Source: CAD feature listing. Evaluate the final solid. Frame: model axes, mm. A direction names the side the tool comes from. Give positions to 0.01 mm unless a question says otherwise; leave off trailing zeros. Loops run counter-clockwise (first coordinate to the right, second up) from the corner with the lowest first, then second, coordinate; pieces in that order, holes last. Notation, with made-up numbers: (-13.5, 88) - (33.5, 88) arc R21 ccw to (33.5, 105) - close; hole circle Ø6 at (66, -5.75). An arc over 180 degrees is marked (long way). Put each result on its own line as item: value.
Solid Edge part; units mm, degrees
sketch "Sketch1" plane through (0, 0, 0) normal (0, -1, 0) x (1, 0, 0)
  line L0 (4.25, 5) -> (4.25, 0)
  line L1 (4.25, 0) -> (2.85, 0)
  line L2 (2.85, 0) -> (2.5, -0.6062)
  line L3 (2.5, -0.6062) -> (2.5, -40)
  line L4 (2.5, -40) -> (0, -40)
  line L5 (2.3, 2.5) -> (0, 1.1721)
  line L6 (2.3, 5) -> (2.3, 2.5)
  line L7 (4.25, 5) -> (2.3, 5)
revolve "RevolvedProtrusion1" add sketch "Sketch1" angle 360 about axis through (0, 0, -6) along (0, 0, 1)
cosmetic_thread "Thread1"
chamfer "Chamfer_1" distance 0.25 angle 45 1 edges at (-2.5, 0, -40)
fillet "Round_1" radius 0.3 2 edges at (-4.25, 0, 0) (-4.25, 0, 5)
sketch "Sketch2" plane through (0, 0, 5) normal (0, 0, 1) x (0, 1, 0)
  line L0 (-2.3, 1.3279) -> (-2.3, -1.3279)
  line L1 (0, -2.6558) -> (-2.3, -1.3279)
  line L2 (2.3, -1.3279) -> (0, -2.6558)
  line L3 (2.3, 1.3279) -> (2.3, -1.3279)
  line L4 (0, 2.6558) -> (2.3, 1.3279)
  line L5 (-2.3, 1.3279) -> (0, 2.6558)
extrude "Cutout1" cut sketch "Sketch2" against normal up to vertex (2.5 mm away)
properties part number "STD-DIN912-M5x40x8.8" material "Galvanized steel"
1) Material intervals for line 1 along Z through (x, y) = (2.75, 2.25); line 2 along Y through (x, z) = (0, 2); line 3 along X through (y, z) = (1, -15), sorted ascending. Write a range as [from, to].
Check result:
line 1: [0, 5]
line 2: [-4.25, -1.43], [1.43, 4.25]
line 3: [-2.29, 2.29]
2) Pin query (flat end, axial travel): P1, Ø2, axis at x = 1, z = -24.5, coming from the -Y side; P2, Ø1.3, axis at x = -1, y = 1.5, coming from the +Z side; P3, Ø1.3, axis at x = -1, y = -2, coming from the +Z side; P4, Ø1.5, axis at x = 0, y = -0.5, coming from the +Z side. Return the tip coordinate at first contact, or that it passes through.
Check result:
P1: y = -2.5
P2: z = 2.5
P3: z = 5
P4: z = 1.89
3) Mould query, pull axis X, two halves, no side actions, for faces 3 (the cylindrical face through (2.285, -3.584, 2.469)), 4 (the flat face through (1, -3, 0)), 5 (the conical face through (-0.087, -0.39, 1.403)). Classes: pulls with the +X half, pulls with the -X half, needs draft (parallel to the pull), parting line crosses it, or undercut.
Check result:
face 3: parting line crosses it
face 4: needs draft
face 5: undercut
4) Access query for faces 1 (the flat face through (2, -2, 5)), 2 (the flat face through (1.663, -1.719, 3.768)). Directions: +Z, -Z, +X, -X, +Y, -Y. A direction counts if a zero-diameter tool reaches every point of the face in a straight line with its end or side. Return the directions, or none.
Check result:
face 1: +Z, +X, -X, +Y, -Y
face 2: +Z
5) Section query A-A, the plane z = -20.5. Output: boundary loops of the cut face in (x, y).
Check result:
outline: circle Ø5 at (0, 0)
